```python
from build123d import *

# Parameters (mm, degrees)
SKETCH1_R           = 100
BOSS_EXTRUDE1_DEPTH = 10
SKETCH4_R           = 1.73
CUT_EXTRUDE2_DEPTH  = 11
SKETCH6_R           = 1.75
CUT_EXTRUDE3_DEPTH  = 10
SKETCH7_R           = 3
CUT_EXTRUDE4_DEPTH  = 3.5
CUT_EXTRUDE5_DEPTH  = 5.1
CUT_EXTRUDE6_DEPTH  = 5.1
SKETCH10_R          = 1.75
CUT_EXTRUDE7_DEPTH  = 5.9
CUT_EXTRUDE9_DEPTH  = 5.1
SKETCH13_R          = 1.75
CUT_EXTRUDE10_DEPTH = 5.9
CUT_EXTRUDE11_DEPTH = 11
CUT_EXTRUDE12_DEPTH = 11
SKETCH18_R          = 2.75
CUT_EXTRUDE13_DEPTH = 5.9


with BuildPart() as part:
    # Sketch1 → Boss-Extrude1 (new body)
    with BuildSketch(Plane(origin=(0, 0, 0), x_dir=(1, 0, 0), z_dir=(0, 1, 0))):
        Circle(SKETCH1_R)
    extrude(amount=BOSS_EXTRUDE1_DEPTH)

    # Sketch4 → Cut-Extrude2 (cut, through all)
    with BuildSketch(Plane(origin=(0, 10, 0), x_dir=(1, 0, 0), z_dir=(0, 1, 0))):
        with Locations((-82.085, 0)):
            Circle(SKETCH4_R)
        with Locations((0, -36.5)):
            Circle(SKETCH4_R)
        with Locations((82.085, 0)):
            Circle(SKETCH4_R)
        with Locations((0, 36.5)):
            Circle(SKETCH4_R)
    extrude(amount=-CUT_EXTRUDE2_DEPTH, mode=Mode.SUBTRACT)

    # Sketch6 → Cut-Extrude3 (cut)
    with BuildSketch(Plane.XZ):
        with Locations((8, 0)):
            Circle(SKETCH6_R)
        with Locations((0, 9.5)):
            Circle(SKETCH6_R)
        with Locations((-8, 0)):
            Circle(SKETCH6_R)
        with Locations((0, -9.5)):
            Circle(SKETCH6_R)
    extrude(amount=-CUT_EXTRUDE3_DEPTH, mode=Mode.SUBTRACT)

    # Sketch7 → Cut-Extrude4 (cut)
    with BuildSketch(Plane(origin=(0, 10, 0), x_dir=(1, 0, 0), z_dir=(0, 1, 0))):
        with Locations((0, 9.5)):
            Circle(SKETCH7_R)
        with Locations((-8, 0)):
            Circle(SKETCH7_R)
        with Locations((0, -9.5)):
            Circle(SKETCH7_R)
        with Locations((8, 0)):
            Circle(SKETCH7_R)
    extrude(amount=-CUT_EXTRUDE4_DEPTH, mode=Mode.SUBTRACT)

    # Sketch8 → Cut-Extrude5 (cut)
    with BuildSketch(Plane(origin=(0, 10, 0), x_dir=(1, 0, 0), z_dir=(0, 1, 0))):
        with BuildLine():
            Line((-14.3, -79.8), (-14.3, -99.17434144))
            ThreePointArc((-14.3, -99.17434144), (-20.033793367, -98.17681561), (-25.7, -96.848076904))
            Line((-25.7, -96.848076904), (-25.7, -79.8))
            Line((-25.7, -79.8), (-14.3, -79.8))
        make_face()
        with BuildLine():
            Line((25.7, -79.8), (25.7, -96.848076904))
            ThreePointArc((25.7, -96.848076904), (20.033793367, -98.17681561), (14.3, -99.17434144))
            Line((14.3, -99.17434144), (14.3, -79.8))
            Line((14.3, -79.8), (25.7, -79.8))
        make_face()
    extrude(amount=-CUT_EXTRUDE5_DEPTH, mode=Mode.SUBTRACT)

    # Sketch9 → Cut-Extrude6 (cut)
    with BuildSketch(Plane(origin=(0, 10, 0), x_dir=(1, 0, 0), z_dir=(0, 1, 0))):
        with BuildLine():
            Line((-12.9, 99.164459359), (-12.9, 89.8))
            Line((-12.9, 89.8), (12.9, 89.8))
            Line((12.9, 89.8), (12.9, 99.164459359))
            ThreePointArc((12.9, 99.164459359), (0, 100), (-12.9, 99.164459359))
        make_face()
    extrude(amount=-CUT_EXTRUDE6_DEPTH, mode=Mode.SUBTRACT)

    # Sketch10 → Cut-Extrude7 (cut, through all)
    with BuildSketch(Plane(origin=(0, 4.9, 0), x_dir=(1, 0, 0), z_dir=(0, 1, 0))):
        with Locations((-7.7, 94.48222968)):
            Circle(SKETCH10_R)
        with Locations((7.7, 94.48222968)):
            Circle(SKETCH10_R)
    extrude(amount=-CUT_EXTRUDE7_DEPTH, mode=Mode.SUBTRACT)

    # Sketch12 → Cut-Extrude9 (cut)
    with BuildSketch(Plane(origin=(0, 10, 0), x_dir=(1, 0, 0), z_dir=(0, 1, 0))):
        with BuildLine():
            Line((67.079669869, 74.433580394), (59.821233688, 67.175144213))
            Line((59.821233688, 67.175144213), (67.175144213, 59.821233688))
            Line((67.175144213, 59.821233688), (74.433580394, 67.079669869))
            ThreePointArc((74.433580394, 67.079669869), (70.852099475, 70.852099475), (67.079669869, 74.433580394))
        make_face()
    cut_extrude9 = extrude(amount=-CUT_EXTRUDE9_DEPTH, mode=Mode.SUBTRACT)

    # Sketch13 → Cut-Extrude10 (cut, through all)
    with BuildSketch(Plane(origin=(0, 4.9, 0), x_dir=(1, 0, 0), z_dir=(0, 1, 0))):
        with Locations((67.175144213, 67.175144213)):
            Circle(SKETCH13_R)
    cut_extrude10 = extrude(amount=-CUT_EXTRUDE10_DEPTH, mode=Mode.SUBTRACT)

    # Mirror1: Cut-Extrude9, Cut-Extrude10 across plane
    add(cut_extrude9.mirror(Plane(origin=(0, 0, 0), x_dir=(0, 0, 1), z_dir=(1, 0, 0))), mode=Mode.SUBTRACT)
    add(cut_extrude10.mirror(Plane(origin=(0, 0, 0), x_dir=(0, 0, 1), z_dir=(1, 0, 0))), mode=Mode.SUBTRACT)

    # Sketch15 → Cut-Extrude11 (cut, through all)
    with BuildSketch(Plane(origin=(0, 10, 0), x_dir=(1, 0, 0), z_dir=(0, 1, 0))):
        with BuildLine():
            Line((-22.984410516, -49.967157946), (-41.789837303, -90.849378084))
            ThreePointArc((-41.789837303, -90.849378084), (-67.258268931, -74.002197673), (-86.455078863, -50.254545455))
            Line((-86.455078863, -50.254545455), (-47.550293374, -27.64))
            ThreePointArc((-47.550293374, -27.64), (-36.992047912, -40.70120872), (-22.984410516, -49.967157946))
        make_face()
        with BuildLine():
            Line((22.984410516, -49.967157946), (41.789837303, -90.849378084))
            ThreePointArc((41.789837303, -90.849378084), (67.258268931, -74.002197673), (86.455078863, -50.254545455))
            Line((86.455078863, -50.254545455), (47.550293374, -27.64))
            ThreePointArc((47.550293374, -27.64), (36.992047912, -40.70120872), (22.984410516, -49.967157946))
        make_face()
    extrude(amount=-CUT_EXTRUDE11_DEPTH, mode=Mode.SUBTRACT)

    # Sketch17 → Cut-Extrude12 (cut, through all)
    with BuildSketch(Plane(origin=(0, 10, 0), x_dir=(1, 0, 0), z_dir=(0, 1, 0))):
        with BuildLine():
            Line((-31.784523452, 44.885900558), (-57.79004264, 81.610728288))
            ThreePointArc((-57.79004264, 81.610728288), (-42.108464674, 90.7021345), (-25.043347605, 96.813381))
            Line((-25.043347605, 96.813381), (-13.773841183, 53.24735955))
            ThreePointArc((-13.773841183, 53.24735955), (-23.159655571, 49.886173975), (-31.784523452, 44.885900558))
        make_face()
        with BuildLine():
            Line((13.773841183, 53.24735955), (25.043347605, 96.813381))
            ThreePointArc((25.043347605, 96.813381), (42.108464674, 90.7021345), (57.79004264, 81.610728288))
            Line((57.79004264, 81.610728288), (31.784523452, 44.885900558))
            ThreePointArc((31.784523452, 44.885900558), (23.159655571, 49.886173975), (13.773841183, 53.24735955))
        make_face()
    extrude(amount=-CUT_EXTRUDE12_DEPTH, mode=Mode.SUBTRACT)

    # Sketch18 → Cut-Extrude13 (cut, through all)
    with BuildSketch(Plane(origin=(0, 4.9, 0), x_dir=(1, 0, 0), z_dir=(0, 1, 0))):
        with Locations((-20, -88)):
            Circle(SKETCH18_R)
        with Locations((20, -88)):
            Circle(SKETCH18_R)
    extrude(amount=-CUT_EXTRUDE13_DEPTH, mode=Mode.SUBTRACT)


solid = part.part
```
Geometry: final body of the model. Coordinates: model frame, mm. A direction names the side the tool comes from. Round coordinates to 2 decimals unless told otherwise and drop trailing zeros. Loops run counter-clockwise (first coordinate to the right, second up) from the corner with the lowest first, then second, coordinate; pieces in that order, holes last.
Item 1: Section B-B, the plane x = -72. Output: boundary loops of the cut face in (y, z).
Checked values:
outline: (0, -69.4) - (4.9, -69.4) - (4.9, -64.65) - (10, -64.65) - (10, 41.85) - (0, 41.85) - close
Item 2: Contact query for flat-ended pins moving along their axis: P1, Ø5, axis at x = -47, y = 3.5, coming from the -Z side; P2, Ø3, axis at x = 0.5, z = 8.5, coming from the +Y side; P3, Ø1.5, axis at x = 16.5, y = 7.5, coming from the +Z side. Output: stop coordinate, or through.
Checked values:
P1: stops at z = -69.9
P2: stops at y = 6.5
P3: stops at z = 79.8
Item 3: Line query: L1, parallel to X at y = 7.8, z = 0 (3 decimals); L2, parallel to Z at x = 0, y = 4.25; L3, parallel to X at y = 6.5, z = -55. Output: solid intervals per line, ascending.
Checked values:
L1: x = -100 to -83.815, -80.355 to -11, -5 to 5, 11 to 80.355, 83.815 to 100
L2: z = -100 to -38.23, -34.77 to -11.25, -7.75 to 7.75, 11.25 to 34.77, 38.23 to 100
L3: x = -83.52 to -38.95, -14.23 to 14.23, 38.95 to 83.52
Item 4: Reachability of faces 4 (the flat face through (70.684, 7.486, -63.33)), 5 (the flat face through (67.28, 5.07, 39.11)), 6 (the flat face through (44.969, 5.07, -63.505)), 7 (the flat face through (0, 6.5, -7.5)), 8 (the flat face through (32.255, 5.07, 70.122)) from +Z, -Z, +X, -X, +Y, -Y: full face, straight path, thin tool, end or side. Return the list, or none.
Checked values:
face 4: -Z, +Y
face 5: +Z, +Y, -Y
face 6: -Z, +Y, -Y
face 7: +Y
face 8: +X, +Y, -Y
Item 5: Mould query, pull axis X, two halves, no side actions, for faces 1 (the cylindrical face through (-0.6, 4.9, 100)), 2 (the flat face through (63.447, 7.486, -63.55)), 3 (the flat face through (-1, 0, -1)). Classes: released by +X, released by -X, zero draft, split by the parting line, or undercut.
Checked values:
face 1: split by the parting line
face 2: undercut
face 3: zero draft
Item 6: Section C-C, the plane z = -32.5. Output: boundary loops of the cut face in (x, y).
Checked values:
outline: (-94.57, 0) - (94.57, 0) - (94.57, 10) - (-94.57, 10) - close
Item 7: Section A-A, the plane y = 2. State how many separate pieces and enclosed holes the cut face has, plus the area to 3 significant figures.
Checked values:
separate pieces: 1
enclosed holes: 14
area: 24,400 mm2
